For this review, take the finished solid that the model builds, in its own axes (mm). A direction names the side the tool comes from. Coordinates: 2 decimals unless noted, no trailing zeros. Loops run counter-clockwise (first coordinate to the right, second up) from the corner with the lowest first, then second, coordinate; pieces in that order, holes last. Notation, with made-up numbers: M 28,46.5 L 37,46.5 A15 cw 37,74.5 Z; hole C -37.75,41.5 d10. An arc over 180 degrees is marked long. Answer as a JSON object with one key per item and string values. Group by question number.
Item 1: Wall thickness on L1, parallel to Z at x = 0, y = 4; L2, parallel to Z at x = 0, y = 2; L3, parallel to X at y = 6, z = -4.75: over which ranges is each line inside the solid? List them lowest first. Write a range as from..to.
Item 2: Tool access review of faces 5 (the face through (1, 7, -2)), 6 (the face through (0.715, 3.549, 1.375)): name each direction out of +Z, -Z, +X, -X, +Y, -Y from which nothing blocks a thin tool from reaching the whole face with its end or side.
Item 3: Add section B-B (z = 0). State the section outline as (x, y) points, then the cut area to 3 significant figures.
Item 4: Add section A-A (x = 0). State the section outline as (y, z) points, then the cut area to 3 significant figures.
Item 5: Insertion check: pin 1 (3 mm diameter, centred on x = 2.5, y = 11, fed in from +Z); pin 2 (5 mm diameter, centred on x = 0, z = 0, fed in from -Y); pin 3 (1 mm diameter, centred on x = 6, y = 8, fed in from -Z) (3 decimals); pin 4 (1 mm diameter, centred on y = 4, z = -7, fed in from +X). Each pin has a flat end and moves straight along its axis. Give the tip position at first contact, or say it passes through.
Item 6: Mouldability with a two-part tool opening along Y and no side actions: class faces 1 (the face through (-1.19, 10.97, -5.37)), 2 (the face through (3, 0, 0)), 3 (the face through (6, 13, 0)), 4 (the face through (11.923, 6.553, -3.755)) as +Y half, -Y half, draft (parallel to the pull), parting line (faces both ways), or undercut.
Autodesk Inventor part; units mm, degrees
ref_plane "YZ Plane" through (0, 0, 0) normal (1, 0, 0) x (0, 1, 0)
ref_plane "XZ Plane" through (0, 0, 0) normal (0, 1, 0) x (-1, 0, 0)
ref_plane "XY Plane" through (0, 0, 0) normal (0, 0, 1) x (1, 0, 0)
sketch "Szkic1" plane through (0, 0, 0) normal (0, 0, 1) x (1, 0, 0)
  line L0 (0, 0) -> (13.5, 0)
  line L1 (13.5, 0) -> (13.5, 1)
  line L2 (13.5, 1) -> (12.5, 1)
  line L3 (12.5, 1) -> (12.5, 12)
  line L4 (12.5, 12) -> (13.5, 12)
  line L5 (13.5, 12) -> (13.5, 13)
  line L6 (13.5, 13) -> (5.5, 13)
  line L7 (5.5, 13) -> (5.5, 7)
  line L8 (5.5, 7) -> (3.1, 7)
  line L9 (3.1, 7) -> (0, 7)
  line L10 (0, 7) -> (0, 0)
  dimension "d0" = 13.5
  dimension "d1" = 1
  dimension "d2" = 1
  dimension "d3" = 11
  dimension "d4" = 1
  dimension "d5" = 1
  dimension "d6" = 8
  dimension "d7" = 6
  dimension "d8" = 2.4
revolve "Obrót1" add sketch "Szkic1" angle 360 about axis through (0, 7, 0) along (0, -1, 0)
sketch "Szkic2" plane through (0, 7, 0) normal (0, 1, 0) x (1, 0, 0)
  circle A0 centre (0, 0) radius 5.5
  circle A1 centre (0, 0) radius 1.55
  dimension "d10" = 3.1
extrude "Wyciągnięcie proste1" cut sketch "Szkic2" against normal blind 10 contours A1
fillet "Zaokrąglenie1" radius 2 3 edges at (-12.5, 1, 0) (-12.5, 12, 0) (-5.5, 7, 0)
properties part number "Kolo"
From the geometry:
{
 "1": {"L1": "z = -12.5..-1.55, 1.55..12.5", "L2": "z = -12.64..-1.55, 1.55..12.64", "L3": "x = -11.56..11.56"},
 "2": {"face 5": "+Y", "face 6": "+Y, -Y"},
 "3": {"outline": "M -13.5,0 L -1.55,0 L -1.55,7 L -3.5,7 A2 cw -5.5,9 L -5.5,13 L -13.5,13 L -13.5,12 A2 cw -12.5,10.27 L -12.5,2.73 A2 cw -13.5,1 Z; M 1.55,0 L 13.5,0 L 13.5,1 A2 cw 12.5,2.73 L 12.5,10.27 A2 cw 13.5,12 L 13.5,13 L 5.5,13 L 5.5,9 A2 cw 3.5,7 L 1.55,7 Z", "area": "245 mm²"},
 "4": {"outline": "M 0,-13.5 L 1,-13.5 A2 cw 2.73,-12.5 L 10.27,-12.5 A2 cw 12,-13.5 L 13,-13.5 L 13,-5.5 L 9,-5.5 A2 cw 7,-3.5 L 7,-1.55 L 0,-1.55 Z; M 0,1.55 L 7,1.55 L 7,3.5 A2 cw 9,5.5 L 13,5.5 L 13,13.5 L 12,13.5 A2 cw 10.27,12.5 L 2.73,12.5 A2 cw 1,13.5 L 0,13.5 Z", "area": "245 mm²"},
 "5": {"pin 1": "stops at z = 13.43", "pin 2": "stops at y = 0", "pin 3": "stops at z = -11.225", "pin 4": "stops at x = 10.68"},
 "6": {"face 1": "draft", "face 2": "-Y half", "face 3": "+Y half", "face 4": "undercut"}
}
